Autodesk Inventor part; units mm, degrees
ref_plane "YZ Plane" through (0, 0, 0) normal (1, 0, 0) x (0, 1, 0)
ref_plane "XZ Plane" through (0, 0, 0) normal (0, 1, 0) x (-1, 0, 0)
ref_plane "XY Plane" through (0, 0, 0) normal (0, 0, 1) x (1, 0, 0)
sketch "Sketch1" plane through (0, 0, 0) normal (0, 0, 1) x (1, 0, 0)
  line L0 (0, 0) -> (170, 0)
  line L1 (170, 0) -> (170, 310)
  line L2 (170, 310) -> (0, 310)
  line L3 (0, 310) -> (0, 0)
  dimension "d0" = 310
  dimension "d1" = 170
extrude "Extrusion1" add sketch "Sketch1" along normal blind 150
sketch "Sketch2" plane through (0, 0, 150) normal (0, 0, 1) x (1, 0, 0)
  line L0 (20, 290) -> (150, 290)
  line L1 (150, 290) -> (150, 20)
  line L2 (150, 20) -> (20, 20)
  line L3 (20, 20) -> (20, 290)
  line L4 (170, 310) -> (0, 310)
  line L5 (0, 310) -> (0, 0)
  line L6 (0, 0) -> (170, 0)
  line L7 (170, 0) -> (170, 310)
  dimension "d4" = 20
  dimension "d5" = 20
  dimension "d6" = 20
  dimension "d7" = 20
sketch "Sketch3" plane through (0, 310, 0) normal (0, 1, 0) x (1, 0, 0)
  line L0 (20, -20) -> (150, -20)
  line L1 (150, -20) -> (150, -130)
  line L2 (150, -130) -> (20, -130)
  line L3 (20, -130) -> (20, -20)
  line L4 (170, 0) -> (0, 0)
  line L5 (0, 0) -> (0, -150)
  line L6 (170, -150) -> (0, -150)
  line L7 (170, 0) -> (170, -150)
  dimension "d8" = 20
  dimension "d9" = 20
  dimension "d10" = 20
  dimension "d11" = 20
sketch "Sketch4" plane through (170, 0, 0) normal (1, 0, 0) x (0, 0, -1)
  line L0 (-130, 290) -> (-20, 290)
  line L1 (-20, 290) -> (-20, 20)
  line L2 (-20, 20) -> (-130, 20)
  line L3 (-130, 20) -> (-130, 290)
  line L4 (0, 310) -> (-150, 310)
  line L5 (-150, 0) -> (-150, 310)
  line L6 (0, 0) -> (-150, 0)
  line L7 (0, 0) -> (0, 310)
  dimension "d12" = 20
  dimension "d13" = 20
  dimension "d14" = 20
  dimension "d15" = 20
extrude "Extrusion2" cut sketch "Sketch4" against normal blind 900 contours L0 L1 L2 L3
extrude "Extrusion3" cut sketch "Sketch2" against normal blind 900 contours L0 L1 L2 L3
extrude "Extrusion4" cut sketch "Sketch3" against normal blind 40 contours L0 L1 L2 L3
sketch "Sketch5" plane through (170, 0, 0) normal (1, 0, 0) x (0, 0, -1)
  line L0 (-150, 0) -> (-150, 310)
  line L1 (-150, 310) -> (0, 310)
  line L2 (0, 310) -> (0, 135)
  line L3 (0, 135) -> (-150, 135)
  line L4 (-150, 135) -> (-150, 310)
  point P0 (0, 0)
  point P1 (-150, 135)
  dimension "d22" = 175
extrude "Extrusion5" cut sketch "Sketch5" against normal through all
sketch "Sketch6" plane through (0, 0, 150) normal (0, 0, 1) x (1, 0, 0)
  line L0 (20, 135) -> (0, 135)
  line L1 (0, 135) -> (20, 135)
  line L2 (20, 135) -> (20, 20)
  line L3 (0, 20) -> (0, 135)
  line L4 (0, 0) -> (170, 0)
  line L5 (0, 0) -> (170, 0)
  line L6 (170, 0) -> (170, 20)
  line L7 (0, 20) -> (0, 0)
  line L8 (150, 135) -> (170, 135)
  line L9 (170, 135) -> (170, 20)
  line L10 (150, 20) -> (150, 135)
  line L11 (20, 20) -> (150, 20)
  line L12 (20, 20) -> (150, 20)
extrude "Extrusion6" add sketch "Sketch6" along normal blind 10
sketch "Sketch7" plane through (170, 20, 130) normal (1, 0, 0) x (0, 0, -1)
  line L0 (0, 115) -> (-30, 115)
  line L1 (-30, 0) -> (0, 0)
  line L2 (0, 115) -> (-10, 115)
  line L3 (-10, 115) -> (-10, 0)
  line L4 (-10, 0) -> (0, 0)
  line L5 (0, 0) -> (0, 115)
  point P0 (130, -20)
  point P1 (-10, 115)
  dimension "d27" = 10
extrude "Extrusion7" cut sketch "Sketch7" against normal through all
sketch "Sketch8" plane through (0, 20, 20) normal (0, 0, 1) x (1, 0, 0)
  line L0 (20, 115) -> (20, 0)
  line L1 (0, 115) -> (20, 115)
  line L2 (20, 115) -> (20, 95)
  line L3 (20, 95) -> (0, 95)
  line L4 (0, 95) -> (0, 115)
  point P0 (0, -20)
  dimension "d30" = 20
sketch "Sketch9" plane through (150, 20, 20) normal (0, 0, 1) x (1, 0, 0)
  line L0 (20, 115) -> (20, 0)
  line L1 (20, 115) -> (0, 115)
  line L2 (0, 115) -> (0, 95)
  line L3 (0, 95) -> (20, 95)
  line L4 (20, 95) -> (20, 115)
  point P0 (-150, -20)
  point P1 (20, 95)
  dimension "d31" = 20
extrude "Extrusion8" add sketch "Sketch8" along normal up to surface (120 mm away)
extrude "Extrusion9" add sketch "Sketch9" along normal up to surface (120 mm away)
sketch "Sketch10" plane through (0, 135, 0) normal (0, 1, 0) x (1, 0, 0)
  line L0 (0, -160) -> (0, 0)
  line L1 (20, 0) -> (20, -160)
  line L2 (0, 0) -> (20, 0)
  line L3 (20, 0) -> (20, -160)
  line L4 (20, -160) -> (0, -160)
  line L5 (0, -160) -> (0, 0)
  line L6 (0, 0) -> (170, 0)
  line L7 (150, -140) -> (150, -160)
  line L8 (170, 0) -> (150, 0)
  line L9 (150, 0) -> (150, -160)
  line L10 (150, -160) -> (170, -160)
  line L11 (170, -160) -> (170, 0)
  point P0 (150, 0)
extrude "Extrusion10" add sketch "Sketch10" along normal blind 10
sketch "Sketch11" plane through (170, 0, 160) normal (1, 0, 0) x (0, 0, -1)
  line L0 (140, 115) -> (20, 115)
  line L1 (20, 115) -> (140, 115)
  line L2 (140, 115) -> (140, 125)
  line L3 (140, 125) -> (20, 125)
  line L4 (20, 125) -> (20, 115)
  point P0 (160, 0)
  dimension "d38" = 10
extrude "Extrusion11" cut sketch "Sketch11" against normal through all
sketch "Sketch12" plane through (0, 145, 0) normal (0, 1, 0) x (1, 0, 0)
  line L0 (20, -160) -> (20, -140)
  line L1 (0, 0) -> (20, 0)
  line L2 (20, 0) -> (20, -160)
  line L3 (20, -160) -> (0, -160)
  line L4 (0, -160) -> (0, 0)
  line L5 (170, 0) -> (170, -160)
  line L6 (170, 0) -> (150, 0)
  line L7 (150, 0) -> (150, -160)
  line L8 (150, -160) -> (170, -160)
  line L9 (170, -160) -> (170, 0)
extrude "Extrusion12" add sketch "Sketch12" along normal blind 5
sketch "Sketch13" plane through (170, 0, 160) normal (1, 0, 0) x (0, 0, -1)
  line L0 (20, 125) -> (140, 125)
  line L1 (20, 125) -> (140, 125)
  line L2 (140, 125) -> (140, 130)
  line L3 (140, 130) -> (20, 130)
  line L4 (20, 130) -> (20, 125)
  point P0 (160, 0)
  dimension "d43" = 5
extrude "Extrusion13" cut sketch "Sketch13" against normal through all
sketch "Sketch14" plane through (0, 150, 0) normal (0, 1, 0) x (1, 0, 0)
  line L0 (20, -160) -> (20, -140)
  line L1 (0, 0) -> (20, 0)
  line L2 (20, 0) -> (20, -160)
  line L3 (20, -160) -> (0, -160)
  line L4 (0, -160) -> (0, 0)
  line L5 (0, 0) -> (170, 0)
  line L6 (150, -160) -> (20, -160)
  line L7 (170, 0) -> (150, 0)
  line L8 (150, 0) -> (150, -160)
  line L9 (150, -160) -> (170, -160)
  line L10 (170, -160) -> (170, 0)
extrude "Extrusion14" add sketch "Sketch14" along normal blind 5 contours L3 L4 L1 L2 L0 | L8 L5 L10 L9
sketch "Sketch15" plane through (170, 0, 160) normal (1, 0, 0) x (0, 0, -1)
  line L0 (20, 130) -> (140, 130)
  line L1 (20, 130) -> (140, 130)
  line L2 (140, 130) -> (140, 135)
  line L3 (140, 135) -> (20, 135)
  line L4 (20, 135) -> (20, 130)
  point P0 (160, 0)
  dimension "d48" = 5
extrude "Extrusion15" cut sketch "Sketch15" against normal through all
sketch "Sketch17" plane through (0, 0, 0) normal (0, 0, -1) x (-1, 0, 0)
  line L0 (0, 155) -> (-20, 155)
  line L1 (0, 155) -> (-20, 155)
  line L2 (-20, 155) -> (-20, 135)
  line L3 (-20, 135) -> (0, 135)
  line L4 (0, 135) -> (0, 155)
  point P0 (0, 0)
  dimension "d52" = 20
extrude "Extrusion16" add sketch "Sketch17" along normal blind 25.003
sketch "Sketch18" plane through (20, 20, 20) normal (1, 0, 0) x (0, 0, -1)
  line L0 (-140, 135) -> (20, 135)
  line L1 (-120, 115) -> (0, 115)
  line L2 (-140, 135) -> (-120, 135)
  line L3 (-120, 135) -> (-120, 115)
  line L4 (-120, 115) -> (-140, 115)
  line L5 (-140, 115) -> (-140, 135)
  point P0 (20, -20)
  point P1 (-120, 135)
extrude "Extrusion17" add sketch "Sketch18" along normal up to surface (130 mm away)
properties part number "Pump and motor housing new"
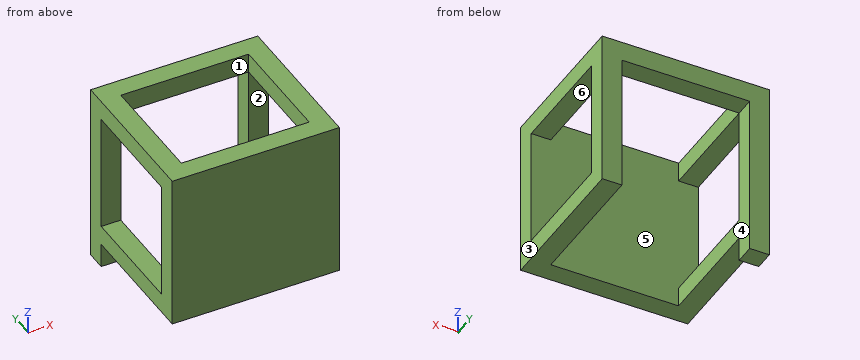
Geometry: final body of the model. Coordinates: model frame, mm. Face numbers are marked on the shaded views. A direction names the side the tool comes from. Round coordinates to 2 decimals unless told otherwise and drop trailing zeros. Loops run counter-clockwise (first coordinate to the right, second up) from the corner with the lowest first, then second, coordinate; pieces in that order, holes last.
Item 1: Section B-B, the plane x = 17.5. Output: boundary loops of the cut face in (y, z), plus the area to 3 significant figures.
Checked values:
outline: (0, 0) - (135, 0) - (135, -25) - (155, -25) - (155, 160) - (0, 160) - close; hole (20, 20) - (135, 20) - (135, 140) - (20, 140) - close
area: 11,500 mm2
Item 2: Mould query, pull axis X, two halves, no side actions, for the marked faces 1, 2 and 3. Classes: released by +X, released by -X, zero draft, split by the parting line, or undercut.
Checked values:
face 1: undercut
face 2: zero draft
face 3: released by +X
Item 3: Contact query for flat-ended pins moving along their axis: P1, Ø10, axis at x = 156.5, y = 74.5, coming from the -Z side; P2, Ø4, axis at x = 78.5, z = 101.5, coming from the +Y side; P3, Ø10, axis at x = 82.5, y = 145.5, coming from the -Z side. Output: stop coordinate, or through.
Checked values:
P1: stops at z = 0
P2: stops at y = 20
P3: stops at z = 140
Item 4: Line query: L1, parallel to Z at x = 12, y = 47.5; L2, parallel to X at y = 37, z = 7.5; L3, parallel to Z at x = 95, y = 137.5. Output: solid intervals per line, ascending.
Checked values:
L1: z = 0 to 20, 140 to 160
L2: x = 0 to 20, 150 to 170
L3: z = 140 to 160
Item 5: Section C-C, the plane y = 63.5. Output: boundary loops of the cut face in (x, z), plus the area to 3 significant figures.
Checked values:
outline: (0, 0) - (20, 0) - (20, 20) - (0, 20) - close; (0, 140) - (20, 140) - (20, 160) - (0, 160) - close; (150, 0) - (170, 0) - (170, 20) - (150, 20) - close; (150, 140) - (170, 140) - (170, 160) - (150, 160) - close
area: 1,600 mm2
Item 6: Section A-A, the plane z = 25. Output: boundary loops of the cut face in (x, y).
Checked values:
outline: (0, 0) - (170, 0) - (170, 20) - (0, 20) - close; (0, 135) - (20, 135) - (20, 155) - (0, 155) - close; (150, 135) - (170, 135) - (170, 155) - (150, 155) - close
Item 7: Section D-D, the plane x = 39.5. Output: boundary loops of the cut face in (y, z).
Checked values:
outline: (0, 0) - (20, 0) - (20, 160) - (0, 160) - close; (135, 140) - (155, 140) - (155, 160) - (135, 160) - close
Item 8: Reachability of the marked faces 4, 5 and 6 from +Z, -Z, +X, -X, +Y, -Y: full face, straight path, thin tool, end or side. Return the list, or none.
Checked values:
face 4: -Z, +Y
face 5: none
face 6: +X, -X
